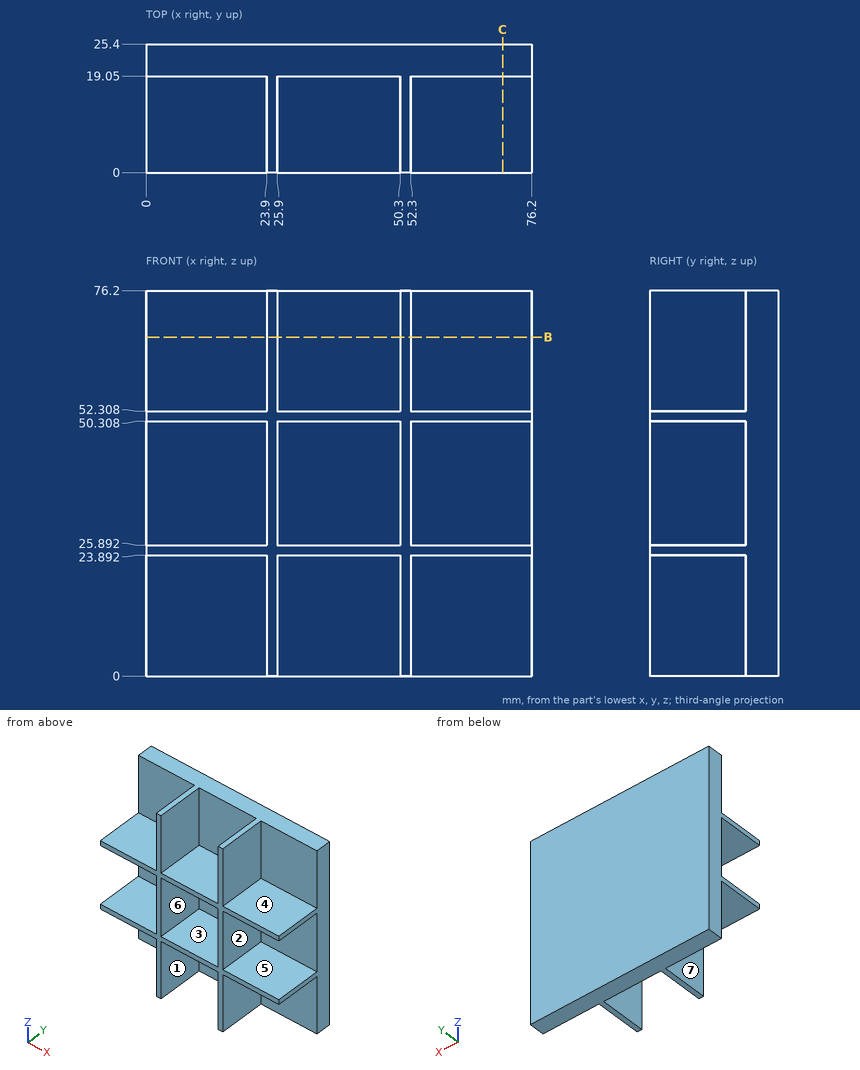
Geometry check sheet. Reference: drawing and pictorial views, mm from the part's lowest x, y, z. A direction names the side the tool comes from. Coordinates: 2 decimals unless noted, no trailing zeros. Write each loop counter-clockwise with the first axis right and the second up, starting at its lowest first coordinate (ties: lowest second). Pieces come first, ordered by that corner, then holes. Notation, with made-up numbers: M 87,-7.75 L 99,-7.75 A22 ccw 99,28.25 Z; hole C 43,75.5 d6. An arc over 180 degrees is marked long. Use one line per item in the form item = value.
Item 1: Material ranges on L1, parallel to X at y = 4, z = 11; L2, parallel to Z at x = 56, y = 8.75; L3, parallel to Y at x = 61, z = 35.5, recorded low to high. Write a range as from..to.
Answer below:
L1 = 23.9..25.9, 50.3..52.3
L2 = 23.89..25.89, 50.31..52.31
L3 = 19.05..25.4
Item 2: Set-up check for the marked faces 1, 2, 3 and 4: record each of +Z, -Z, +X, -X, +Y, -Y from which the full face is reachable in a straight line by a thin tool's end or side.
Answer below:
face_1 = -Z, -Y
face_2 = +X, -Y
face_3 = -Y
face_4 = +Z, +X, -Y
Item 3: Gauge pin test, flat ends, axial feed: pin 1 Ø5.5 at (x, y) = (40.5, 10.5) entering from -Z; pin 2 Ø9.5 at (y, z) = (13, 62) entering from +X; pin 3 Ø12 at (x, z) = (66, 8.5) entering from -Y. Record the tip position at first contact, or that the pin passes through.
Answer below:
pin_1 = 23.89
pin_2 = 52.3
pin_3 = 19.05
Item 4: Sectioned sample at C-C, the plane x = 70.5. Record the cut outline in (y, z).
Answer below:
outline = M 0,23.89 L 19.05,23.89 L 19.05,0 L 25.4,0 L 25.4,76.2 L 19.05,76.2 L 19.05,52.31 L 0,52.31 L 0,50.31 L 19.05,50.31 L 19.05,25.89 L 0,25.89 Z
Item 5: Release check for a two-part mould opening along X. For the marked faces 5, 6 and 7 record: pulls with the +X half, pulls with the -X half, needs draft (parallel to the pull), parting line crosses it, or undercut.
Answer below:
face_5 = needs draft
face_6 = undercut
face_7 = pulls with the -X half
Item 6: Sectioned sample at B-B, the plane z = 67. Record the cut outline in (x, y).
Answer below:
outline = M 0,19.05 L 23.9,19.05 L 23.9,0 L 25.9,0 L 25.9,19.05 L 50.3,19.05 L 50.3,0 L 52.3,0 L 52.3,19.05 L 76.2,19.05 L 76.2,25.4 L 0,25.4 Z
